Could you check a few things on this model? Use its own coordinates, in mm. Give positions to 0.01 mm unless a question says otherwise; leave off trailing zeros. Order: outer loops, then holes, each group sorted by start corner. A loop starts at its lowest first (then second) coordinate and runs counter-clockwise, first axis right, second up. Notation, with made-up numbers: (25.25, -10.75) - (50.25, -10.75) arc R17 cw to (50.25, 16.25) - close; hole circle Ø1 at (4, 21). An arc over 180 degrees is marked (long way). One line per question, with ' | ' between items. Start each with the question number.
1. Imagine slicing it at B-B (z = -31). Please give me the cut outline in (x, y).
2. Imagine slicing it at C-C (x = -64). Please give me the cut outline in (y, z).
3. For P1, Ø0.5, axis at y = 5, z = 76, coming from the +X side; P2, Ø5, axis at y = 3, z = 18.5, coming from the +X side; P3, Ø2.5, axis at x = 73.025, z = 0, coming from the +Y side; P4, Ø3, axis at y = 4.5, z = 0, coming from the +X side, each with a flat end and sliding along its axis, tell me the tip position at first contact or that it passes through.
4. Imagine slicing it at A-A (y = 2.5). Give the number of separate pieces and of enclosed holes in the cut face, and give its area (3 significant figures).
5. I need wall thicknesses on probe 1 along X at (y, z) = (5, 0); probe 2 along Z at (x, y) = (51.5, 2); probe 3 along Z at (x, y) = (1, 7.5). Which ranges of each line are inside material? Lowest first, please. Write a range as from..to.
```python
from build123d import *

# Parameters (mm, degrees)
SKETCH2_R                = 76.2
BOSS_EXTRUDE1_DEPTH      = 12.7
BOSS_EXTRUDE2_DEPTH      = 78.74
BOSS_EXTRUDE2_DEPTH_BACK = 78.74
FILLET1_R                = 2.54
SKETCH4_R                = 1.50114
CUT_EXTRUDE1_DEPTH       = 111.307377813


with BuildPart() as part:
    # Sketch2 → Boss-Extrude1 (new body)
    with BuildSketch(Plane(origin=(0, 0, 0), x_dir=(1, 0, 0), z_dir=(0, 1, 0))):
        with Locations(Location((0, 0, 0), (0, 0, 270))):
            Circle(SKETCH2_R)
    extrude(amount=BOSS_EXTRUDE1_DEPTH)

    # Sketch3 → Boss-Extrude2 (add, two sides: drawn at the far end of the back side and taken through both)
    with BuildSketch(Plane.XY.offset(-BOSS_EXTRUDE2_DEPTH_BACK)):
        Polygon((0, 0), (-19.05, 0), (-19.05, 12.7), (19.05, 12.7), (19.05, 0), align=None)
    extrude(amount=BOSS_EXTRUDE2_DEPTH + BOSS_EXTRUDE2_DEPTH_BACK)

    # Fillet1
    fillet1_edges = [part.edges().sort_by_distance(p)[0] for p in [
        (-19.05, 6.35, -78.74),
        (19.05, 6.35, -78.74),
        (-19.05, 6.35, -73.780332745),
        (-19.05, 6.35, 73.780332745),
        (19.05, 6.35, 73.780332745),
        (19.05, 6.35, -73.780332745),
        (19.05, 6.35, 78.74),
        (-19.05, 6.35, 78.74),
    ]]
    fillet(fillet1_edges, radius=FILLET1_R)

    # Sketch4 → Cut-Extrude1 (cut, through all)
    with BuildSketch(Plane(origin=(0, 12.7, 0), x_dir=(1, 0, 0), z_dir=(0, 1, 0))):
        with Locations(Location((73.025, 0, 0), (0, 0, 270))):
            Circle(SKETCH4_R)
        with Locations(Location((51.636472696, -51.636472696, 0), (0, 0, 270))):
            Circle(SKETCH4_R)
        with Locations(Location((0, -73.025, 0), (0, 0, 270))):
            Circle(SKETCH4_R)
        with Locations(Location((-51.636472696, -51.636472696, 0), (0, 0, 270))):
            Circle(SKETCH4_R)
        with Locations(Location((-73.025, 0, 0), (0, 0, 270))):
            Circle(SKETCH4_R)
        with Locations(Location((-51.636472696, 51.636472696, 0), (0, 0, 270))):
            Circle(SKETCH4_R)
        with Locations(Location((0, 73.025, 0), (0, 0, 270))):
            Circle(SKETCH4_R)
        with Locations(Location((51.636472696, 51.636472696, 0), (0, 0, 270))):
            Circle(SKETCH4_R)
    extrude(amount=-CUT_EXTRUDE1_DEPTH, mode=Mode.SUBTRACT)


solid = part.part
```
Results found:
1) outline: (-69.61, 0) - (69.61, 0) - (69.61, 12.7) - (-69.61, 12.7) - close
2) outline: (0, -41.36) - (12.7, -41.36) - (12.7, 41.36) - (0, 41.36) - close
3) P1: stops at x = 19.05 | P2: stops at x = 74.5 | P3: passes through | P4: stops at x = 76.2
4) separate pieces: 1 | enclosed holes: 8 | area: 18,400 mm2
5) probe 1: x = -76.2..-74.53, -71.52..71.52, 74.53..76.2 | probe 2: z = -56.16..-53.13, -50.14..50.14, 53.13..56.16 | probe 3: z = -78.74..-74.14, -71.91..71.91, 74.14..78.74
